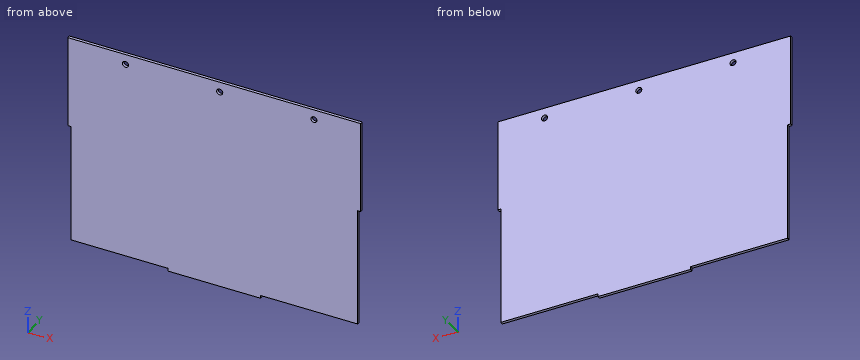
from build123d import *

# Parameters (mm, degrees)
SKETCH1_W           = 315.58
SKETCH1_H           = 3.175
BOSS_EXTRUDE1_DEPTH = 232.600000128
SKETCH5_W           = 3.175
SKETCH5_H           = 130.999992
CUT_EXTRUDE2_DEPTH  = 282.088108579
SKETCH7_R           = 3.302
CUT_EXTRUDE3_DEPTH  = 282.088108579
LPATTERN1_COUNT     = 3
LPATTERN1_PITCH     = 101.6
SKETCH10_W          = 99.68
SKETCH10_H          = 3.175
BOSS_EXTRUDE2_DEPTH = 3.175


with BuildPart() as part:
    # Sketch1 → Boss-Extrude1 (new body)
    with BuildSketch(Plane.XY):
        Rectangle(SKETCH1_W, SKETCH1_H)
    extrude(amount=BOSS_EXTRUDE1_DEPTH)

    # Sketch5 → Cut-Extrude2 (cut, symmetric)
    with BuildSketch(Plane(origin=(0, 1.5875, 0), x_dir=(1, 0, 0), z_dir=(0, 1, 0))):
        with Locations((-156.2025, -65.499996)):
            Rectangle(SKETCH5_W, SKETCH5_H)
    cut_extrude2 = extrude(amount=CUT_EXTRUDE2_DEPTH, both=True, mode=Mode.SUBTRACT)

    # Mirror1: Cut-Extrude2 across plane
    add(cut_extrude2.mirror(Plane(origin=(0, 0, 0), x_dir=(0, 0, 1), z_dir=(1, 0, 0))), mode=Mode.SUBTRACT)

    # Sketch7 → Cut-Extrude3 (cut, through all)
    with BuildSketch(Plane.XZ.offset(1.5875)):
        with Locations(Location((107.495393219, 221.30835, 0), (0, 0, 270))):
            Circle(SKETCH7_R)
    cut_extrude3 = extrude(amount=-CUT_EXTRUDE3_DEPTH, mode=Mode.SUBTRACT)

    # LPattern1: Cut-Extrude3 ×3
    with Locations(*[(-i * LPATTERN1_PITCH, 0, 0) for i in range(1, LPATTERN1_COUNT)]):
        add(cut_extrude3, mode=Mode.SUBTRACT)

    # Sketch10 → Boss-Extrude2 (add)
    with BuildSketch(Plane(origin=(0, 0, 0), x_dir=(-1, 0, 0), z_dir=(0, 0, -1))):
        Rectangle(SKETCH10_W, SKETCH10_H)
    extrude(amount=BOSS_EXTRUDE2_DEPTH)


solid = part.part
The model under review builds one solid part; all positions refer to its coordinate system, in mm. Round coordinates to 2 decimals unless told otherwise and drop trailing zeros. Order: outer loops, then holes, each group sorted by start corner. A loop starts at its lowest first (then second) coordinate and runs counter-clockwise, first axis right, second up. Notation, with made-up numbers: (32.5, -39.5) -> (67.5, -39.5) arc R13 cw to (67.5, -35.5) -> close; hole circle Ø6 at (44.5, 30). An arc over 180 degrees is marked (long way). Write item = value, one per line. Start each with the question number.
Item 1: Consider section A-A on y = 0.8. Write out the cut boundary in (x, z) (3 decimals).
Item 2: Clearance check with flat-ended pins moving along their axes: pin 1 Ø1 at (y, z) = (-0.5, 88.5) entering from -X (3 decimals); pin 2 Ø1 at (x, y) = (-107.5, -0.5) entering from -Z; pin 3 Ø1.6 at (y, z) = (1, -1) entering from +X. State where each tip first meets the part, or that it passes through.
Item 3: Consider section B-B on z = 58. Write out the cut boundary in (x, y) (1 decimal), plus the area to 3 significant figures.
Item 4: For line 1 along Z through (x, y) = (126.5, 0.5); line 2 along X through (y, z) = (0.35, 22) (3 decimals); line 3 along Z through (x, y) = (4, 0.3) (3 decimals), list the stretches that pass through material, from the lowest coordinate up.
Conclusion:
q1.outline = (-157.79, 131) -> (-154.615, 131) -> (-154.615, 0) -> (-49.84, 0) -> (-49.84, -3.175) -> (49.84, -3.175) -> (49.84, 0) -> (154.615, 0) -> (154.615, 131) -> (157.79, 131) -> (157.79, 232.6) -> (-157.79, 232.6) -> close; hole circle Ø6.604 at (-95.705, 221.308); hole circle Ø6.604 at (5.895, 221.308); hole circle Ø6.604 at (107.495, 221.308)
q2.pin_1 = -154.615
q2.pin_2 = 0
q2.pin_3 = 49.84
q3.outline = (-154.6, -1.6) -> (154.6, -1.6) -> (154.6, 1.6) -> (-154.6, 1.6) -> close
q3.area = 982 mm2
q4.line_1 = 0 to 232.6
q4.line_2 = -154.615 to 154.615
q4.line_3 = -3.175 to 218.605, 224.012 to 232.6
